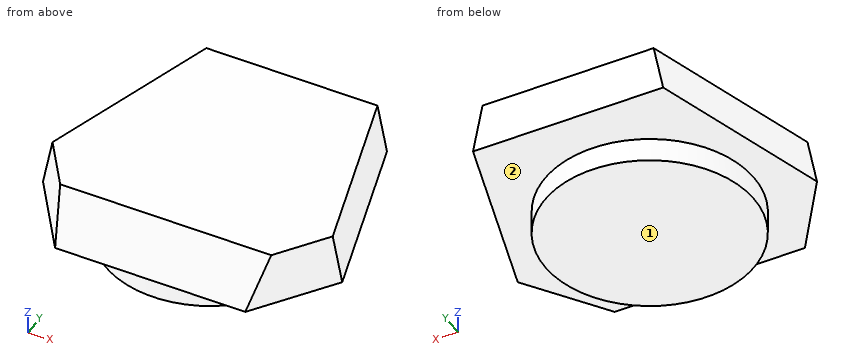
from build123d import *

# Parameters (mm, degrees)
F4_R     = 27.7189698501
F5_DEPTH = 6.35


with BuildPart() as f3:
    # F0 (on Top) → F3 section 0
    with BuildSketch(Plane.XY):
        Polygon((-25.4, -20.8064619249), (0, -20.8064619249), (25.4, -20.8064619249), (39.9688414833, 0), (25.4, 48.666095568), (0, 48.666095568), (-25.4, 48.666095568), (-39.9688414833, 0), align=None)
    # F2 (on offset) → F3 section 1
    with BuildSketch(Plane.XY.offset(12.7)):
        Polygon((22.86, 48.6660952), (0, 48.6660952), (-22.86, 48.6660952), (-37.4288413732, 0), (-28.195581331, -13.1864619249), (0, -13.1864619249), (28.1955748, -13.1864619249), (37.4288348422, 0), align=None)
    loft()

    # F4 (on face) → F5 (join)
    with BuildSketch(Plane(origin=(0, 0, 0), x_dir=(1, 0, 0), z_dir=(0, 0, -1))):
        with Locations((0, -8.6576407775)):
            Circle(F4_R)
    extrude(amount=F5_DEPTH)


solid = f3.part
Read the model definition and answer for the solid it produces. Units are mm, in the model's axes. Face numbers are marked on the shaded views. A direction names the side the tool comes from. Round coordinates to 2 decimals unless told otherwise and drop trailing zeros. Order: outer loops, then holes, each group sorted by start corner. A loop starts at its lowest first (then second) coordinate and runs counter-clockwise, first axis right, second up.
1) The part is cut by section A-A on z = -4. Write down the section's boundary in (x, y), plus the area to 3 significant figures.
2) Straight lines are drawn through the part: L1, parallel to Z at x = 24, y = -9; L2, parallel to X at y = 19.5, z = -3; L3, parallel to Y at x = -7.5, z = 6.5. For each, find the intervals that lie inside material, in ascending order.
3) Flat-ended cylindrical pins translate along their axes: pin 1 (1.5 mm diameter, centred on y = 30.5, z = 8.5, fed in from +X); pin 2 (8 mm diameter, centred on x = -10, z = -2, fed in from -Y); pin 3 (5 mm diameter, centred on x = 28.5, z = 0.5, fed in from -Y). Find the tip coordinate at first contact, or state that the pin passes through.
4) For the marked faces 1 and 2, determine the directions among +Z, -Z, +X, -X, +Y, -Y from which every point of the face is accessible in a straight line to the end or side of a thin tool.
Resolved:
1. outline: circle Ø55.44 at (0, 8.66)
1. area: 2,410 mm2
2. L1: z = 0 to 12.7
2. L2: x = -25.51 to 25.51
2. L3: y = -16.91 to 48.67
3. pin 1: stops at x = 29.41
3. pin 2: stops at y = -20.81
3. pin 3: stops at y = -19.88
4. face 1: -Z, +X, -X, +Y, -Y
4. face 2: -Z
